Source: three-view drawing plus pictorial views. Frame: mm from the lowest corner of the part. A direction names the side the tool comes from. Give positions to 0.01 mm unless a question says otherwise; leave off trailing zeros. Loops run counter-clockwise (first coordinate to the right, second up) from the corner with the lowest first, then second, coordinate; pieces in that order, holes last. Notation, with made-up numbers: M 74,-32 L 109,-32 A32 cw 109,6 Z; hole C -39,25.5 d1. An arc over 180 degrees is marked long. Answer as a JSON object with one key per item and string values. Group by question number.
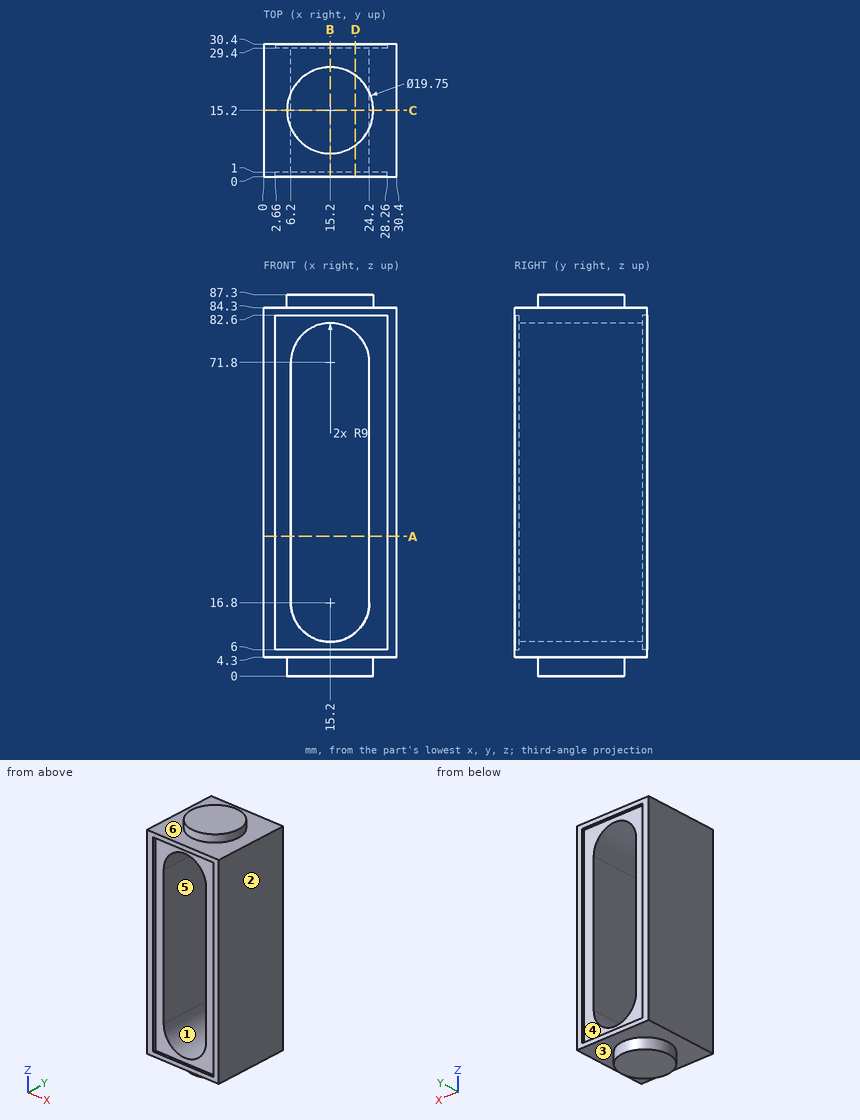
1. Mould query, pull axis X, two halves, no side actions, for the marked faces 1, 2 and 3. Classes: pulls with the +X half, pulls with the -X half, needs draft (parallel to the pull), parting line crosses it, or undercut.
2. Section A-A (z = 32). Output: boundary loops of the cut face in (x, y), then the cut area to 3 significant figures.
3. First-contact query: P1, Ø1.1, axis at x = 15.5, y = 30, coming from the -Z side; P2, Ø0.8, axis at x = 10.5, y = 0.5, coming from the +Z side; P3, Ø12, axis at x = 21, z = 30.5, coming from the +Y side. Flat tips, straight axial feed; report the tip coordinate or a pass-through.
4. Reachability of the marked faces 4, 5 and 6 from +Z, -Z, +X, -X, +Y, -Y: full face, straight path, thin tool, end or side. Return the list, or none.
5. Section C-C (y = 15.2). Output: boundary loops of the cut face in (x, z) (1 decimal), then the cut area to 3 significant figures.
6. Section B-B (x = 15.2). Output: boundary loops of the cut face in (y, z) (1 decimal).
7. Section D-D (x = 21). Output: boundary loops of the cut face in (y, z).
8. Material intervals for L1, parallel to Z at x = 15, y = 17; L2, parallel to X at y = 13.5, z = 26.5; L3, parallel to Y at x = 26.5, z = 81, sorted ascending.
Geometry results:
{
 "1": {"face 1": "undercut", "face 2": "pulls with the +X half", "face 3": "needs draft"},
 "2": {"outline": "M 0,0 L 2.66,0 L 2.66,1 L 6.2,1 L 6.2,29.4 L 2.66,29.4 L 2.66,30.4 L 0,30.4 Z; M 24.2,1 L 28.26,1 L 28.26,0 L 30.4,0 L 30.4,30.4 L 28.26,30.4 L 28.26,29.4 L 24.2,29.4 Z", "area": "362 mm2"},
 "3": {"P1": "z = 4.3", "P2": "z = 84.3", "P3": "y = 29.4"},
 "4": {"face 4": "+Y", "face 5": "+Y, -Y", "face 6": "+Z"},
 "5": {"outline": "M 0,4.3 L 5.3,4.3 L 5.3,0 L 25.1,0 L 25.1,4.3 L 30.4,4.3 L 30.4,84.3 L 25.1,84.3 L 25.1,87.3 L 5.3,87.3 L 5.3,84.3 L 0,84.3 Z; hole M 6.2,16.8 A9 ccw 24.2,16.8 L 24.2,71.8 A9 ccw 6.2,71.8 Z", "area": "1,330 mm2"},
 "6": {"outline": "M 0,4.3 L 5.3,4.3 L 5.3,0 L 25.1,0 L 25.1,4.3 L 30.4,4.3 L 30.4,6 L 29.4,6 L 29.4,7.8 L 1,7.8 L 1,6 L 0,6 Z; M 0,82.6 L 1,82.6 L 1,80.8 L 29.4,80.8 L 29.4,82.6 L 30.4,82.6 L 30.4,84.3 L 25.1,84.3 L 25.1,87.3 L 5.3,87.3 L 5.3,84.3 L 0,84.3 Z"},
 "7": {"outline": "M 0,4.3 L 7.21,4.3 L 7.21,0 L 23.19,0 L 23.19,4.3 L 30.4,4.3 L 30.4,6 L 29.4,6 L 29.4,9.92 L 1,9.92 L 1,6 L 0,6 Z; M 0,82.6 L 1,82.6 L 1,78.68 L 29.4,78.68 L 29.4,82.6 L 30.4,82.6 L 30.4,84.3 L 23.19,84.3 L 23.19,87.3 L 7.21,87.3 L 7.21,84.3 L 0,84.3 Z"},
 "8": {"L1": "0 to 7.8, 80.8 to 87.3", "L2": "0 to 6.2, 24.2 to 30.4", "L3": "1 to 29.4"}
}
